Could you check a few things on this drawing? It's one solid part, dimensions in mm from its lowest x, y, z. Round coordinates to 2 decimals unless told otherwise and drop trailing zeros. Order: outer loops, then holes, each group sorted by start corner. A loop starts at its lowest first (then second) coordinate and runs counter-clockwise, first axis right, second up. Notation, with made-up numbers: (0, 78.5) - (5, 78.5) arc R31 cw to (5, 107.5) - close; hole circle Ø6 at (-5, 75.25). An arc over 180 degrees is marked (long way). Use one line per item in the form item = value.
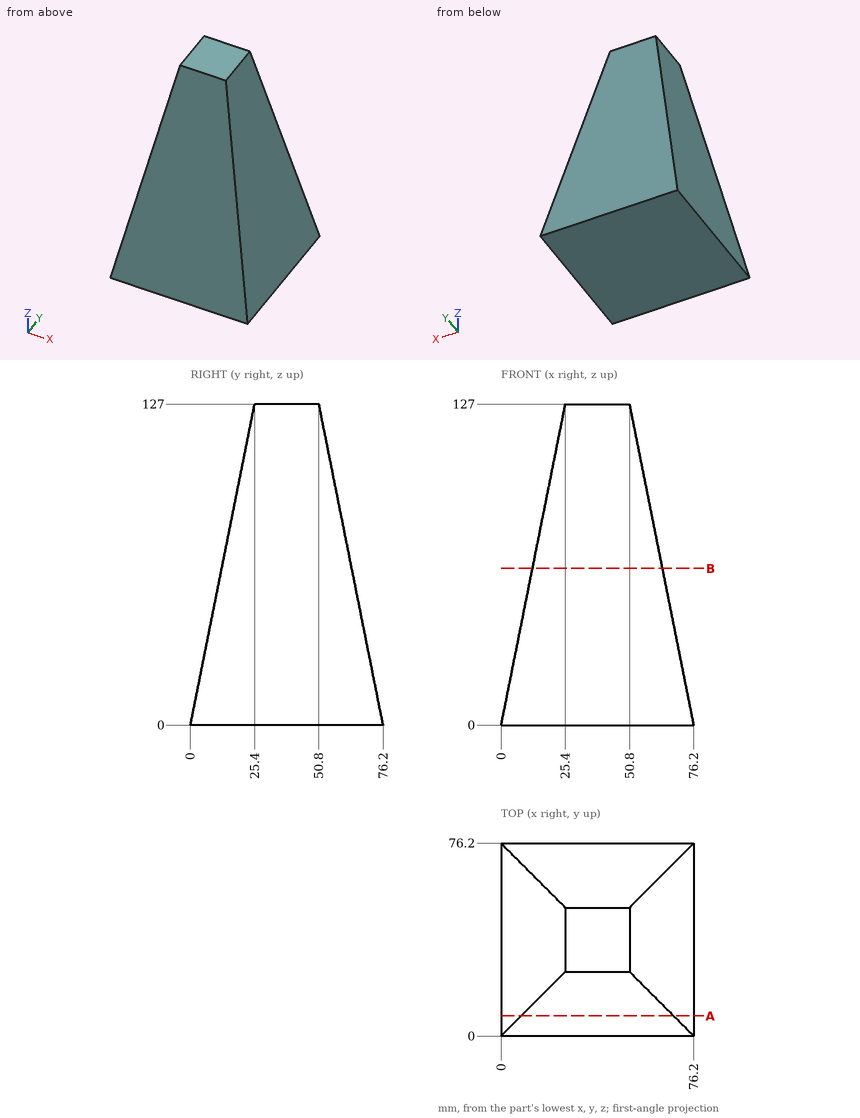
Item 1: I need wall thicknesses on L1, parallel to Y at x = 35, z = 62.5; L2, parallel to X at y = 57.5, z = 33; L3, parallel to X at y = 55, z = 50.5. Which ranges of each line are inside material? Lowest first, please.
Found:
L1 = 12.5 to 63.7
L2 = 6.6 to 69.6
L3 = 10.1 to 66.1
Item 2: Imagine slicing it at A-A on y = 8. Please give me the cut outline in (x, z), plus the area to 3 significant figures.
Found:
outline = (0, 0) - (76.2, 0) - (68.2, 40) - (8, 40) - close
area = 2,730 mm2
Item 3: Will these pins go through, and if not, where does the flat tip stop? P1, Ø10, axis at x = 45, z = 113, coming from the -Y side; P2, Ø3, axis at y = 15, z = 61.5, coming from the +X side; P3, Ø10, axis at x = 49, z = 101.5, coming from the -Y side.
Found:
P1 = 21.6
P2 = 64.2
P3 = 19.3
Item 4: Imagine slicing it at B-B on z = 62. Please give me the cut outline in (x, y), plus the area to 3 significant figures.
Found:
outline = (12.4, 12.4) - (63.8, 12.4) - (63.8, 63.8) - (12.4, 63.8) - close
area = 2,640 mm2
